Could you check a few things on this model? Use its own coordinates, in mm. Round coordinates to 2 decimals unless told otherwise and drop trailing zeros. Loops run counter-clockwise (first coordinate to the right, second up) from the corner with the lowest first, then second, coordinate; pieces in that order, holes last. Notation, with made-up numbers: (51, -20) -> (100, -20) arc R21 ccw to (100, -12) -> close; hole circle Ø5 at (28, 81.25). An arc over 180 degrees is marked (long way). One line per item, written item: value.
```python
from build123d import *

# Parameters (mm, degrees)
EXTRUDE1_DEPTH          = 19.05
EXTRUDE1_DEPTH_BACK     = 19.05
SKETCH1_R               = 2.0828
SKETCH8_OUTSIDE_W       = 152.724
SKETCH8_OUTSIDE_H       = 153.706
SKETCH8_OUTSIDE_R       = 3.175
EXTRUDE4_DEPTH          = 39.407440143
EXTRUDE4_DRAFT          = -60
MIRROR1_COPY_1_SKETCH_W = 152.724
MIRROR1_COPY_1_SKETCH_H = 153.706
MIRROR1_COPY_1_SKETCH_R = 3.175
MIRROR1_COPY_1_DEPTH    = 39.407440143
MIRROR1_COPY_1_DRAFT    = -60


with BuildPart() as part:
    # Sketch1 → Extrude1 (new, two sides: drawn at the far end of the back side and taken through both)
    with BuildSketch(Plane.XY.offset(-EXTRUDE1_DEPTH_BACK)):
        Polygon((0, 3.666174209), (-3.175, 1.833087105), (-3.175, -1.833087105), (0, -3.666174209), (3.175, -1.833087105), (3.175, 1.833087105), align=None)
        with Locations(Location((0, 0, 0), (0, 0, 180))):
            Circle(SKETCH1_R, mode=Mode.SUBTRACT)
    extrude(amount=EXTRUDE1_DEPTH + EXTRUDE1_DEPTH_BACK)

    # Extrude3 cone 1 section (through the dimple's axis) → Extrude3 (revolve, cut)
    with BuildSketch(Plane(origin=(0, 0, -19.05), x_dir=(0, 1, 0), z_dir=(1, 0, 0))):
        Polygon((0, 0), (2.1336, 0), (0, 2.28800588), align=None)
    extrude3 = revolve(axis=Axis((0, 0, -19.05), (0, 0, 1)), mode=Mode.SUBTRACT)


with BuildPart() as extrude4_tool:
    # Sketch8 outside → Extrude4 (with draft: the straight prism first)
    with BuildSketch(Plane(origin=(0, 0, -19.05), x_dir=(-1, 0, 0), z_dir=(0, 0, -1))):
        Rectangle(SKETCH8_OUTSIDE_W, SKETCH8_OUTSIDE_H)
        Circle(SKETCH8_OUTSIDE_R, mode=Mode.SUBTRACT)
    extrude(amount=-EXTRUDE4_DEPTH)
    # Extrude4: the draft: its side faces are tilted about the plane it starts from
    extrude4_sides = [extrude4_tool.faces().sort_by_distance(p)[0] for p in [
        (0, -76.853, 0.653720071),
        (-76.362, 0, 0.653720071),
        (0, 76.853, 0.653720071),
        (76.362, 0, 0.653720071),
        (3.175, 0, 0.653720071),
    ]]
    draft(extrude4_sides, Plane(origin=(0, 0, -19.05), x_dir=(-1, 0, 0), z_dir=(0, 0, -1)), EXTRUDE4_DRAFT)


with BuildPart() as part_1:
    add(part.part)

    # Extrude4: cut by extrude4_tool
    add(extrude4_tool.part, mode=Mode.SUBTRACT)

    # Mirror1: Extrude3 across plane
    add(extrude3.mirror(Plane.XY), mode=Mode.SUBTRACT)


with BuildPart() as mirror1_copy_1_tool:
    # Mirror1 copy 1 sketch → Mirror1 copy 1 (with draft: the straight prism first)
    with BuildSketch(Plane(origin=(0, 0, 19.05), x_dir=(-1, 0, 0), z_dir=(0, 0, 1))):
        Rectangle(MIRROR1_COPY_1_SKETCH_W, MIRROR1_COPY_1_SKETCH_H)
        Circle(MIRROR1_COPY_1_SKETCH_R, mode=Mode.SUBTRACT)
    extrude(amount=-MIRROR1_COPY_1_DEPTH)
    # Mirror1 copy 1: the draft: its side faces are tilted about the plane it starts from
    mirror1_copy_1_sides = [mirror1_copy_1_tool.faces().sort_by_distance(p)[0] for p in [
        (0, -76.853, -0.653720071),
        (-76.362, 0, -0.653720071),
        (0, 76.853, -0.653720071),
        (76.362, 0, -0.653720071),
        (3.175, 0, -0.653720071),
    ]]
    draft(mirror1_copy_1_sides, Plane(origin=(0, 0, 19.05), x_dir=(-1, 0, 0), z_dir=(0, 0, 1)), MIRROR1_COPY_1_DRAFT)


with BuildPart() as part_2:
    add(part_1.part)

    # Mirror1 copy 1: cut by mirror1_copy_1_tool
    add(mirror1_copy_1_tool.part, mode=Mode.SUBTRACT)


solid = part_2.part
```
Item 1: If we section it at A-A on z = 9: List the corners of the cut face in (x, y) for me (3 decimals), plus the area to 3 significant figures.
Output:
outline: (-3.175, -1.833) -> (0, -3.666) -> (3.175, -1.833) -> (3.175, 1.833) -> (0, 3.666) -> (-3.175, 1.833) -> close; hole circle Ø4.166 at (0, 0)
area: 21.3 mm²
Item 2: I need wall thicknesses on line 1 (X direction, y = 1.5, z = 13.5) (3 decimals); line 2 (X direction, y = -1.25, z = -5) (3 decimals); line 3 (Y direction, x = -1.5, z = 13). Which ranges of each line are inside material? Lowest first, please. Write a range as from..to.
Output:
line 1: x = -3.175..-1.445, 1.445..3.175
line 2: x = -3.175..-1.666, 1.666..3.175
line 3: y = -2.8..-1.45, 1.45..2.8
Item 3: If we mould it in two halves opening along Y, with no side actions, what happens to faces 1 (the face through (-1.987, -0.626, -0.266)), 2 (the face through (2.9, 1.67, 18.95)), 3 (the face through (1.57, -2.76, -0.27)), 4 (the face through (-3.175, 0, 0))? For each: released by +Y, released by -Y, zero draft, split by the parting line, or undercut.
Output:
face 1: undercut
face 2: released by +Y
face 3: released by -Y
face 4: zero draft
Item 4: Will these pins go through, and if not, where does the flat tip stop? pin 1 Ø1.5 at (x, z) = (-2, 2.5) entering from +Y; pin 2 Ø2.5 at (x, y) = (0, 0) entering from -Z; pin 3 Ø2 at (x, z) = (0.5, -2) entering from +Y.
Output:
pin 1: stops at y = 2.94
pin 2: passes through
pin 3: stops at y = 3.67
